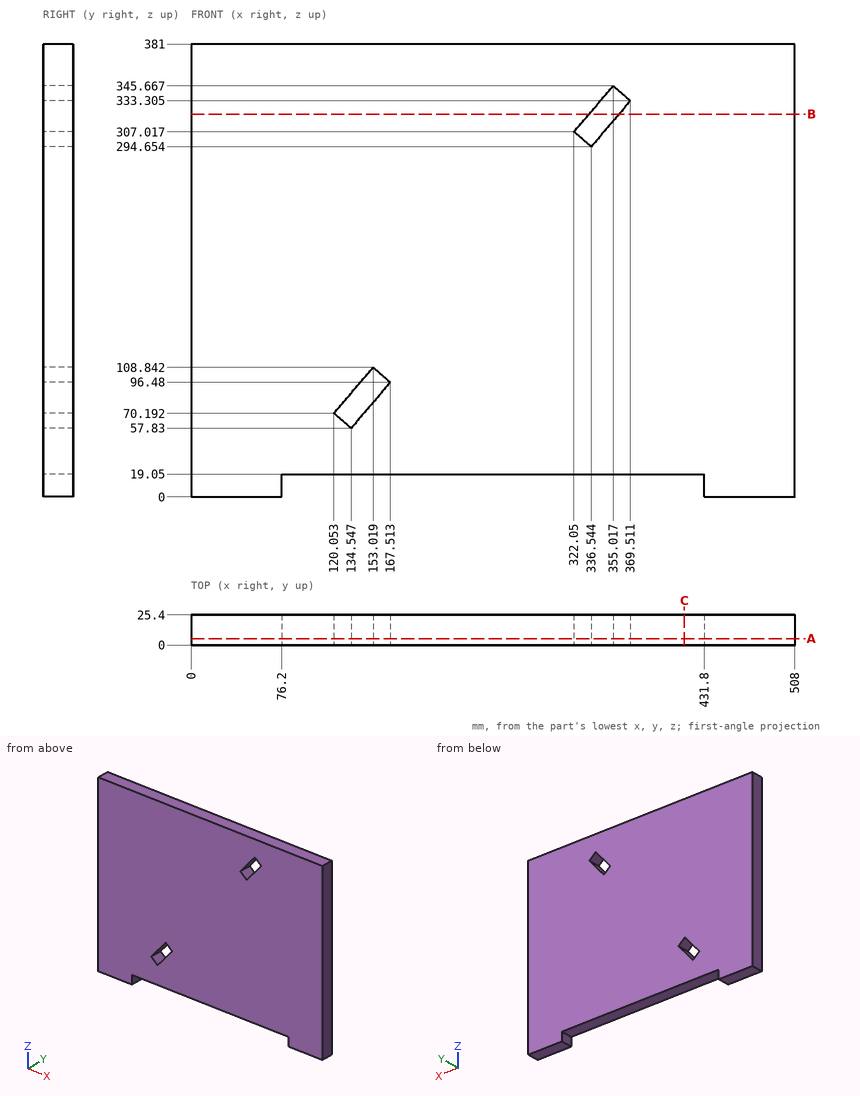
Verification items for this drawing (mm, ordinates from the low corner). Coordinates: 2 decimals unless noted, no trailing zeros. Write each loop counter-clockwise with the first axis right and the second up, starting at its lowest first coordinate (ties: lowest second). Pieces come first, ordered by that corner, then holes. Notation, with made-up numbers: (83, 32.5) - (128, 32.5) arc R21 cw to (128, 41.5) - close; hole circle Ø7 at (77.25, 24.25). An arc over 180 degrees is marked (long way). One line per question, with ' | ' between items.
Item 1: Gauge pin test, flat end, axial feed: P1, Ø12.5, axis at x = 281, y = 12.5, coming from the -Z side. Record the tip position at first contact, or that the pin passes through.
Determined:
P1: stops at z = 19.05
Item 2: Sectioned sample at A-A on y = 5.5. Give the number of separate pieces and of enclosed holes in the cut face, plus the area to 3 significant figures.
Determined:
separate pieces: 1 | enclosed holes: 2 | area: 185,000 mm2
Item 3: Sectioned sample at C-C on x = 415. Record the boundary of the cut face in (y, z).
Determined:
outline: (0, 19.05) - (25.4, 19.05) - (25.4, 381) - (0, 381) - close
Item 4: Sectioned sample at B-B on z = 322. Record the boundary of the cut face in (x, y), plus the area to 3 significant figures.
Determined:
outline: (0, 0) - (334.83, 0) - (334.83, 25.4) - (0, 25.4) - close; (359.87, 0) - (508, 0) - (508, 25.4) - (359.87, 25.4) - close | area: 12,300 mm2
Item 5: Thickness scan on line 1 (X direction, y = 5.5, z = 103) (1 decimal); line 2 (Z direction, x = 275.5, y = 13.25); line 3 (X direction, y = 13.5, z = 325) (1 decimal). Record the ranges inside material, lowest first. Write a range as [from, to].
Determined:
line 1: x = [0, 148], [159.9, 508] | line 2: z = [19.05, 381] | line 3: x = [0, 337.4], [362.4, 508]
